Can you work these out from the model? Positions are in its coordinate system, mm. A direction names the side the tool comes from. Coordinates: 2 decimals unless noted, no trailing zeros. Order: outer loops, then holes, each group sorted by start corner. A loop starts at its lowest first (then second) coordinate and runs counter-clockwise, first axis right, second up. Notation, with made-up numbers: (-9, 79) -> (15, 79) arc R30 cw to (15, 101) -> close; hole circle Ø11 at (38.25, -10.5). An arc over 180 degrees is marked (long way). Use a Markdown table: item, result. Add a question column.
1. We'd pull the mould along Y, two halves only. Please class faces 4 (the flat face through (0, 8, 50)), 5 (the flat face through (13, -20, 98.6)), 6 (the flat face through (17, -47, 50)): pulls with the +Y half, pulls with the -Y half, needs draft (parallel to the pull), parting line crosses it, or undercut.
2. For faces 1 (the flat face through (22, -43, 50)), 2 (the flat face through (22, 3, 50)), 3 (the flat face through (4, -43, 50)), which set-ups out of +Z, -Z, +X, -X, +Y, -Y let a thin tool reach every point of the face, with its end or its side?
3. Suppose I cut it at B-B, the plane z = 1.5. List the corners of the cut face in (x, y) for me, then the cut area to 3 significant figures.
4. Suppose I cut it at A-A, the plane x = 25.25. List the corners of the cut face in (y, z) for me.
5. Suppose I cut it at C-C, the plane y = -36. List the corners of the cut face in (x, z) for me, then the cut area to 3 significant figures.
6. Suppose I cut it at D-D, the plane x = 9.25. List the corners of the cut face in (y, z) for me, then the cut area to 3 significant figures.
7. If I drill on line 1 along Y through (x, z) = (23.75, 1.5); line 2 along Z through (x, y) = (24.75, -17.5); line 3 along Y through (x, z) = (4.5, 50), over which ranges is the centre line in solid material (lowest first)? Write a range as from..to.
8. For pin 1 Ø5 at (x, z) = (21.5, 42.5) entering from -Y; pin 2 Ø1.8 at (x, z) = (-1, 31) entering from -Y; pin 3 Ø1 at (y, z) = (-41.5, 100.5) entering from +X, each with a flat end and sliding along its axis, tell me the tip position at first contact or that it passes through.
Autodesk Inventor part; units mm, degrees
ref_plane "YZ Plane" through (0, 0, 0) normal (1, 0, 0) x (0, 1, 0)
ref_plane "XZ Plane" through (0, 0, 0) normal (0, 1, 0) x (-1, 0, 0)
ref_plane "XY Plane" through (0, 0, 0) normal (0, 0, 1) x (1, 0, 0)
sketch "Sketch2" plane through (0, 0, 0) normal (0, 0, 1) x (1, 0, 0)
  line L0 (-3, 8) -> (-3, -48)
  line L1 (-3, 8) -> (3, 8)
  line L2 (3, 8) -> (3, 3)
  line L3 (3, 3) -> (5, 3)
  line L4 (5, 3) -> (5, 10.4583)
  arc A0 (5, 10.4583) -> (17, 10.4583) centre (11, 13.909) ccw
  line L5 (17, 10.4583) -> (17, 3)
  line L6 (17, 3) -> (27, 3)
  line L7 (-3, -48) -> (3, -48)
  line L8 (3, -43) -> (3, -48)
  line L9 (27, -43) -> (17, -43)
  arc A1 (17, -50.4583) -> (5, -50.4583) centre (11, -53.909) ccw
  line L10 (3, -43) -> (5, -43)
  line L11 (5, -43) -> (5, -50.4583)
  line L12 (17, -43) -> (17, -50.4583)
  line L13 (27, 3) -> (27, 0)
  line L14 (27, 0) -> (0, 0)
  line L15 (0, 0) -> (0, -40)
  line L16 (0, -40) -> (27, -40)
  line L17 (27, -40) -> (27, -43)
  dimension "d13" = 12
  dimension "d14" = 2
  dimension "d20" = 5
  dimension "d22" = 13.843
  dimension "d29" = 3
  dimension "d30" = 3
  dimension "d31" = 3
  dimension "d33" = 40
  dimension "d34" = 27
  dimension "d36" = 16
  dimension "d38" = 67.818
  dimension "d53" = 6.9215
  dimension "d54" = 10
extrude "Extrusion1" add sketch "Sketch2" along normal blind 101.6
sketch "Sketch3" plane through (0, -40, 0) normal (1, 0, 0) x (0, 0, -1)
  line L0 (0, 0) -> (0, 40)
  line L1 (0, 40) -> (-101.6, 40)
  line L2 (-101.6, 0) -> (-101.6, 40)
  line L3 (0, 0) -> (-101.6, 0)
  line L4 (-101.6, 40) -> (-98.6, 40)
  line L5 (-98.6, 40) -> (-98.6, 0)
  line L6 (-98.6, 0) -> (-101.6, 0)
  line L7 (-101.6, 0) -> (-101.6, 40)
  line L8 (0, 40) -> (-3, 40)
  line L9 (-3, 40) -> (-3, 0)
  line L10 (-3, 0) -> (0, 0)
  line L11 (0, 0) -> (0, 40)
  dimension "d39" = 3
  dimension "d40" = 3
extrude "Extrusion2" add sketch "Sketch3" along normal blind 27 contours L3 L9 L1 L0 | L3 L2 L1 L5
sketch "Sketch4" plane through (27, -43, 0) normal (1, 0, 0) x (0, 0, -1)
  circle A0 centre (-100.1, 44.5) radius 1
  line L0 (-3, 3) -> (-98.6, 3)
  line L1 (-98.6, 3) -> (-98.6, 43)
  line L2 (-3, 43) -> (-98.6, 43)
  line L3 (-3, 43) -> (-3, 3)
  line L4 (0, 0) -> (0, 46)
  line L5 (0, 46) -> (-101.6, 46)
  line L6 (-101.6, 0) -> (-101.6, 46)
  line L7 (0, 0) -> (-101.6, 0)
  circle A1 centre (-1.5, 44.5) radius 1
  circle A2 centre (-1.5, 1.5) radius 1
  circle A3 centre (-100.1, 1.5) radius 1
  point P0 (0, 43)
  dimension "d43" = 2
  dimension "d44" = 1.5
  dimension "d45" = 1.5
  dimension "d47" = 1.5
  dimension "d48" = 1.5
extrude "Extrusion3" cut sketch "Sketch4" against normal blind 10 contours A0 | A1 | A2 | A3
equation "\"TUBE_OUTER\" = 13.843"
equation "\"INTER_TUBE\" = 53.975"
equation "\"CUPPING\" = 5.08"
equation "\"d19\" = TUBE_OUTER"
equation "\"W_THICK\" = 3"
equation "\"SCREW_D\" = 2"
properties part number "Casing"
Worked out:
| question | item | result |
|---|---|---|
| 1 | face 4 | pulls with the +Y half |
| 1 | face 5 | undercut |
| 1 | face 6 | needs draft |
| 2 | face 1 | +Z, -Z, +X, -Y |
| 2 | face 2 | +Z, -Z, +X, +Y |
| 2 | face 3 | +Z, -Z, -Y |
| 3 | outline | (-3, -48) -> (3, -48) -> (3, -43) -> (5, -43) -> (5, -50.46) arc R6.92 cw to (17, -50.46) -> (17, -43) -> (27, -43) -> (27, -42.5) -> (17, -42.5) -> (17, -40.5) -> (27, -40.5) -> (27, 0.5) -> (17, 0.5) -> (17, 2.5) -> (27, 2.5) -> (27, 3) -> (17, 3) -> (17, 10.46) arc R6.92 cw to (5, 10.46) -> (5, 3) -> (3, 3) -> (3, 8) -> (-3, 8) -> close |
| 3 | area | 1,520 mm² |
| 4 | outline | (-43, 0) -> (3, 0) -> (3, 101.6) -> (-43, 101.6) -> close; hole circle Ø2 at (-41.5, 1.5); hole circle Ø2 at (-41.5, 100.1); hole (-40, 3) -> (0, 3) -> (0, 98.6) -> (-40, 98.6) -> close; hole circle Ø2 at (1.5, 1.5); hole circle Ø2 at (1.5, 100.1) |
| 5 | outline | (-3, 0) -> (27, 0) -> (27, 3) -> (0, 3) -> (0, 98.6) -> (27, 98.6) -> (27, 101.6) -> (-3, 101.6) -> close |
| 5 | area | 467 mm² |
| 6 | outline | (-47.21, 0) -> (7.21, 0) -> (7.21, 101.6) -> (-47.21, 101.6) -> close; hole (-40, 3) -> (0, 3) -> (0, 98.6) -> (-40, 98.6) -> close |
| 6 | area | 1,710 mm² |
| 7 | line 1 | y = -43..-42.5, -40.5..0.5, 2.5..3 |
| 7 | line 2 | z = 0..3, 98.6..101.6 |
| 7 | line 3 | y = -43..-40, 0..3 |
| 8 | pin 1 | stops at y = -43 |
| 8 | pin 2 | stops at y = -48 |
| 8 | pin 3 | stops at x = 17 |
